Part model, mm, in its own coordinate system. A direction names the side the tool comes from. Round coordinates to 2 decimals unless told otherwise and drop trailing zeros. Order: outer loops, then holes, each group sorted by start corner. A loop starts at its lowest first (then second) coordinate and runs counter-clockwise, first axis right, second up. Notation, with made-up numbers: (65.25, -23) - (96.25, -23) arc R7 ccw to (96.25, -10) - close; hole circle Ø5 at (35.5, -7.5). An arc over 180 degrees is marked (long way). Answer as a JSON object with one key per item and string values.
```python
from build123d import *

# Parameters (mm, degrees)
F0_R     = 10
F1_DEPTH = 1.4
F2_R     = 2.5
F3_DEPTH = 1.4
F5_DEPTH = 2.8
F7_DEPTH = 1.4


with BuildPart() as f1:
    # F0 (on Top) → F1 (new body)
    with BuildSketch(Plane.XY):
        Circle(F0_R)
    extrude(amount=F1_DEPTH)

    # F2 (on face) → F3 (join)
    with BuildSketch(Plane.XY.offset(1.4)):
        Circle(F2_R)
    extrude(amount=F3_DEPTH)

    # F4 (on face) → F5 (join)
    with BuildSketch(Plane.XY.offset(2.8)):
        with BuildLine():
            Line((-2.0478801107, -1.4339410909), (-1.2287280664, -0.8603646545))
            ThreePointArc((-1.2287280664, -0.8603646545), (-1.5, 0), (-1.2287280664, 0.8603646545))
            Line((-1.2287280664, 0.8603646545), (-2.0478801107, 1.4339410909))
            ThreePointArc((-2.0478801107, 1.4339410909), (-2.5, 0), (-2.0478801107, -1.4339410909))
        make_face()
        with BuildLine():
            ThreePointArc((-0.8603646545, 1.2287280664), (0, 1.5), (0.8603646545, 1.2287280664))
            Line((0.8603646545, 1.2287280664), (1.4339410909, 2.0478801107))
            ThreePointArc((1.4339410909, 2.0478801107), (0, 2.5), (-1.4339410909, 2.0478801107))
            Line((-1.4339410909, 2.0478801107), (-0.8603646545, 1.2287280664))
        make_face()
        with BuildLine():
            ThreePointArc((1.2287280664, 0.8603646545), (1.4305754261, 0.4510586993), (1.5, 0))
            ThreePointArc((1.5, 0), (1.4305754261, -0.4510586993), (1.2287280664, -0.8603646545))
            Line((1.2287280664, -0.8603646545), (2.0478801107, -1.4339410909))
            ThreePointArc((2.0478801107, -1.4339410909), (2.3842923769, -0.7517644988), (2.5, 0))
            ThreePointArc((2.5, 0), (2.3842923769, 0.7517644988), (2.0478801107, 1.4339410909))
            Line((2.0478801107, 1.4339410909), (1.2287280664, 0.8603646545))
        make_face()
        with BuildLine():
            Line((1.4339410909, -2.0478801107), (0.8603646545, -1.2287280664))
            ThreePointArc((0.8603646545, -1.2287280664), (0, -1.5), (-0.8603646545, -1.2287280664))
            Line((-0.8603646545, -1.2287280664), (-1.4339410909, -2.0478801107))
            ThreePointArc((-1.4339410909, -2.0478801107), (0, -2.5), (1.4339410909, -2.0478801107))
        make_face()
    extrude(amount=F5_DEPTH)

    # F6 (on face) → F7 (join)
    with BuildSketch(Plane.XY.offset(5.6)):
        with BuildLine():
            ThreePointArc((-0.8603646545, 1.2287280664), (0, 1.5), (0.8603646545, 1.2287280664))
            Line((0.8603646545, 1.2287280664), (1.4339410909, 2.0478801107))
            ThreePointArc((1.4339410909, 2.0478801107), (0, 2.5), (-1.4339410909, 2.0478801107))
            Line((-1.4339410909, 2.0478801107), (-0.8603646545, 1.2287280664))
        make_face()
        with BuildLine():
            ThreePointArc((-1.4339410909, 2.0478801107), (0, 2.5), (1.4339410909, 2.0478801107))
            Line((1.4339410909, 2.0478801107), (1.7207293091, 2.4574561329))
            ThreePointArc((1.7207293091, 2.4574561329), (0, 3), (-1.7207293091, 2.4574561329))
            Line((-1.7207293091, 2.4574561329), (-1.4339410909, 2.0478801107))
        make_face()
        with BuildLine():
            ThreePointArc((3, 0), (2.8611508522, 0.9021173985), (2.4574561329, 1.7207293091))
            Line((2.4574561329, 1.7207293091), (2.0478801107, 1.4339410909))
            Line((2.0478801107, 1.4339410909), (1.2287280664, 0.8603646545))
            ThreePointArc((1.2287280664, 0.8603646545), (1.5, 0), (1.2287280664, -0.8603646545))
            Line((1.2287280664, -0.8603646545), (2.0478801107, -1.4339410909))
            Line((2.0478801107, -1.4339410909), (2.4574561329, -1.7207293091))
            ThreePointArc((2.4574561329, -1.7207293091), (2.8611508522, -0.9021173985), (3, 0))
        make_face()
        with BuildLine():
            Line((-2.0478801107, 1.4339410909), (-2.4574561329, 1.7207293091))
            ThreePointArc((-2.4574561329, 1.7207293091), (-3, 0), (-2.4574561329, -1.7207293091))
            Line((-2.4574561329, -1.7207293091), (-2.0478801107, -1.4339410909))
            ThreePointArc((-2.0478801107, -1.4339410909), (-2.5, 0), (-2.0478801107, 1.4339410909))
        make_face()
        with BuildLine():
            Line((-1.2287280664, 0.8603646545), (-2.0478801107, 1.4339410909))
            ThreePointArc((-2.0478801107, 1.4339410909), (-2.5, 0), (-2.0478801107, -1.4339410909))
            Line((-2.0478801107, -1.4339410909), (-1.2287280664, -0.8603646545))
            ThreePointArc((-1.2287280664, -0.8603646545), (-1.5, 0), (-1.2287280664, 0.8603646545))
        make_face()
        with BuildLine():
            Line((-1.4339410909, -2.0478801107), (-1.7207293091, -2.4574561329))
            ThreePointArc((-1.7207293091, -2.4574561329), (0, -3), (1.7207293091, -2.4574561329))
            Line((1.7207293091, -2.4574561329), (1.4339410909, -2.0478801107))
            Line((1.4339410909, -2.0478801107), (0.8603646545, -1.2287280664))
            ThreePointArc((0.8603646545, -1.2287280664), (0, -1.5), (-0.8603646545, -1.2287280664))
            Line((-0.8603646545, -1.2287280664), (-1.4339410909, -2.0478801107))
        make_face()
    extrude(amount=F7_DEPTH)


solid = f1.part
```
Item 1: Drop flat-ended pins along their axis: P1, Ø4, axis at y = -3.5, z = 5, coming from the -X side; P2, Ø1, axis at x = -1, y = 4, coming from the +Z side. Give the stop position or say it passes through.
Taken from the geometry:
{"P1": "x = -2.54", "P2": "z = 1.4"}
Item 2: Cut at B-B (x = 0). Write the cut outline in (y, z), plus the area to 3 significant figures.
Taken from the geometry:
{"outline": "(-10, 0) - (10, 0) - (10, 1.4) - (2.5, 1.4) - (2.5, 5.6) - (3, 5.6) - (3, 7) - (1.5, 7) - (1.5, 2.8) - (-1.5, 2.8) - (-1.5, 7) - (-3, 7) - (-3, 5.6) - (-2.5, 5.6) - (-2.5, 1.4) - (-10, 1.4) - close", "area": "44.8 mm2"}
Item 3: Cut at A-A (z = 6.5). Write the cut outline in (x, y), plus the area to 3 significant figures.
Taken from the geometry:
{"outline": "(-2.46, -1.72) - (-1.23, -0.86) arc R1.5 cw to (-1.23, 0.86) - (-2.46, 1.72) arc R3 ccw to start; (-1.72, -2.46) arc R3 ccw to (1.72, -2.46) - (0.86, -1.23) arc R1.5 cw to (-0.86, -1.23) - close; (-1.72, 2.46) - (-0.86, 1.23) arc R1.5 cw to (0.86, 1.23) - (1.72, 2.46) arc R3 ccw to start; (1.23, -0.86) - (2.46, -1.72) arc R3 ccw to (2.46, 1.72) - (1.23, 0.86) arc R1.5 cw to start", "area": "16.5 mm2"}
Item 4: Cut at D-D (z = 4.75). Write the cut outline in (x, y), plus the area to 3 significant figures.
Taken from the geometry:
{"outline": "(-2.05, -1.43) - (-1.23, -0.86) arc R1.5 cw to (-1.23, 0.86) - (-2.05, 1.43) arc R2.5 ccw to start; (-1.43, -2.05) arc R2.5 ccw to (1.43, -2.05) - (0.86, -1.23) arc R1.5 cw to (-0.86, -1.23) - close; (-1.43, 2.05) - (-0.86, 1.23) arc R1.5 cw to (0.86, 1.23) - (1.43, 2.05) arc R2.5 ccw to start; (1.23, -0.86) - (2.05, -1.43) arc R2.5 ccw to (2.05, 1.43) - (1.23, 0.86) arc R1.5 cw to start", "area": "9.77 mm2"}
Item 5: Cut at C-C (y = -2.75). Write the cut outline in (x, z), plus the area to 3 significant figures.
Taken from the geometry:
{"outline": "(-9.61, 0) - (9.61, 0) - (9.61, 1.4) - (-9.61, 1.4) - close; (-1.2, 5.6) - (1.2, 5.6) - (1.2, 7) - (-1.2, 7) - close", "area": "30.3 mm2"}
Item 6: Probe L1, parallel to Z at x = -1.25, y = -3; L2, parallel to Y at x = 0.25, z = 6.25; L3, parallel to X at y = 0.5, z = 4.5. List the from-to ranges inside material, lowest first. Write a range as from..to.
Taken from the geometry:
{"L1": "0..1.4", "L2": "-2.99..-1.48, 1.48..2.99", "L3": "-2.45..-1.41, 1.41..2.45"}
Item 7: Two-plate mould, pull along X, no slides. Class faces 1 (the cylindrical face through (0, -3, 6)), 2 (the flat face through (0, 2.7, 5.6)), 3 (the cylindrical face through (-1.5, 0, 4.9)): pulls with the +X half, pulls with the -X half, needs draft (parallel to the pull), parting line crosses it, or undercut.
Taken from the geometry:
{"face 1": "parting line crosses it", "face 2": "needs draft", "face 3": "undercut"}
Item 8: Tool access for faces 4 (the flat face through (0, 0, 2.8)), 5 (the cylindrical face through (-3, 0, 6)), 6 (the cylindrical face through (0, 3, 6)), 7 (the flat face through (-2.7, 0, 5.6)), 8 (the flat face through (2, 0, 7)): list every direction of +Z, -Z, +X, -X, +Y, -Y with a clear straight run to the whole face (end or side of a thin tool).
Taken from the geometry:
{"face 4": "+Z", "face 5": "+Z, -X", "face 6": "+Z, +Y", "face 7": "-X", "face 8": "+Z, +X, -X, +Y, -Y"}
